Could you check a few things on this drawing? It's one solid part, dimensions in mm from its lowest x, y, z. A direction names the side the tool comes from. Give positions to 0.01 mm unless a question says otherwise; leave off trailing zeros. Order: outer loops, then holes, each group sorted by start corner. A loop starts at its lowest first (then second) coordinate and runs counter-clockwise, first axis right, second up. Notation, with made-up numbers: (31, 64) - (70, 64) arc R10 cw to (70, 73) - close; hole circle Ø4 at (-14.75, 39.25). An arc over 180 degrees is marked (long way). Return JSON: item names as keys, results as strings.
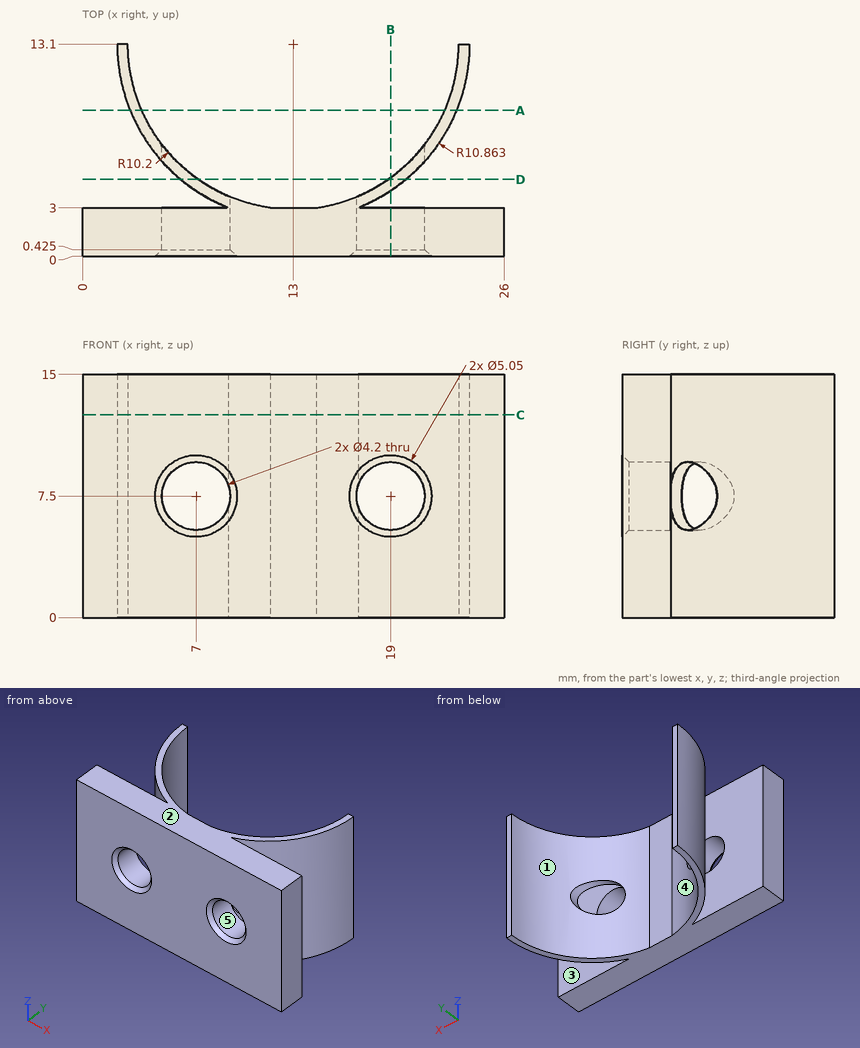
1. Suppose I cut it at B-B (x = 19). List the corners of the cut face in (y, z) for me (1 decimal).
Checks:
{"outline": "(0, 0) - (3, 0) - (3, 5.4) - (0.4, 5.4) - (0, 5) - close; (0, 10) - (0.4, 9.6) - (3, 9.6) - (3, 15) - (0, 15) - close; (4, 0) - (4.9, 0) - (4.9, 5.4) - (4, 5.4) - close; (4, 9.6) - (4.9, 9.6) - (4.9, 15) - (4, 15) - close"}
2. Suppose I cut it at A-A (y = 9). List the corners of the cut face in (x, z) for me, plus the area to 3 significant figures.
Checks:
{"outline": "(2.94, 0) - (3.66, 0) - (3.66, 15) - (2.94, 15) - close; (22.34, 0) - (23.06, 0) - (23.06, 15) - (22.34, 15) - close", "area": "21.6 mm^2"}
3. On a 3-axis mill with a long thin cutter (end or side, diameter ignored), from which of +Z, -Z, +X, -X, +Y, -Y can I reach the whole of each face in a straight line? I mean the marked faces 4 and 5. Say none if no direction works.
Checks:
{"face 4": "+Z, -Z, +Y", "face 5": "+Y, -Y"}
4. If I drill on L1, parallel to Z at x = 7, y = 2.5; L2, parallel to X at y = 0.75, z = 7.75 (3 decimals); L3, parallel to X at y = 0.75, z = 6.75, over which ranges is the centre line in solid material (lowest first)? Write a range as [from, to].
Checks:
{"L1": "[0, 5.4], [9.6, 15]", "L2": "[0, 4.915], [9.085, 16.915], [21.085, 26]", "L3": "[0, 5.04], [8.96, 17.04], [20.96, 26]"}
5. Suppose I cut it at C-C (z = 12.5). List the corners of the cut face in (x, y) for me (1 decimal).
Checks:
{"outline": "(0, 0) - (26, 0) - (26, 3) - (17, 3) arc R10.9 ccw to (23.9, 13.1) - (23.2, 13.1) arc R10.2 cw to (14.4, 3) - (11.6, 3) arc R10.2 cw to (2.8, 13.1) - (2.1, 13.1) arc R10.9 ccw to (9, 3) - (0, 3) - close"}
6. For pin 1 Ø1.4 at (x, z) = (13, 5.5) entering from +Y; pin 2 Ø1 at (y, z) = (10, 4) entering from -X; pin 3 Ø6 at (y, z) = (10.5, 5.5) entering from -X, each with a flat end and sliding along its axis, tell me the tip position at first contact or that it passes through.
Checks:
{"pin 1": "y = 3", "pin 2": "x = 2.45", "pin 3": "x = 2.14"}
7. Thinking about a two-plate mould opening in Y: for the marked faces 1, 2 and 3, which applies, +Y half, -Y half, draft (parallel to the pull), parting line (faces both ways), or undercut?
Checks:
{"face 1": "+Y half", "face 2": "draft", "face 3": "undercut"}
8. Suppose I cut it at D-D (y = 4.75). List the corners of the cut face in (x, z) for me (1 decimal).
Checks:
{"outline": "(6.1, 0) - (7.1, 0) - (7.1, 5.4) arc R2.1 cw to (6.1, 5.6) - close; (6.1, 9.4) arc R2.1 cw to (7.1, 9.6) - (7.1, 15) - (6.1, 15) - close; (18.9, 0) - (19.9, 0) - (19.9, 5.6) arc R2.1 cw to (18.9, 5.4) - close; (18.9, 9.6) arc R2.1 cw to (19.9, 9.4) - (19.9, 15) - (18.9, 15) - close"}
